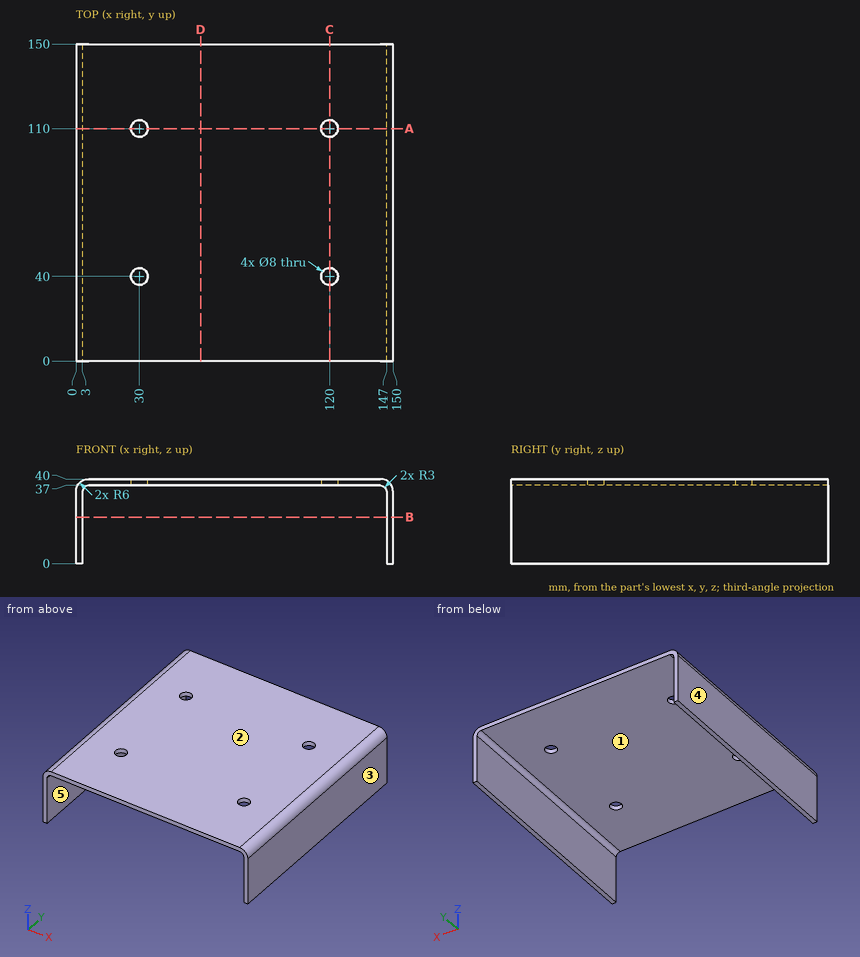
Print and shaded views of the part. All mm, measured from the part's lowest x, y and z. A direction names the side the tool comes from. Give positions to 0.01 mm unless a question says otherwise; leave off trailing zeros. Loops run counter-clockwise (first coordinate to the right, second up) from the corner with the lowest first, then second, coordinate; pieces in that order, holes last. Notation, with made-up numbers: (-13.75, 24) - (-2.75, 24) arc R29 cw to (-2.75, 61) - close; hole circle Ø3 at (35.25, 44.25). An arc over 180 degrees is marked (long way). One line per item, written item: value. Start each with the question number.
1. Which spindle directions (+Z, -Z, +X, -X, +Y, -Y) get a long thin tool onto all of the face, cutting with end or side? Do the marked faces 4 and 5. Say none if no direction does.
2. Pin check, flat tips, straight feed: pin 1 (6.5 mm diameter, centred on x = 30, y = 110, fed in from +Z) (3 decimals); pin 2 (3 mm diameter, centred on x = 113.5, y = 115, fed in from -Z). Stop position of each tip, or through.
3. Slice it at B-B (z = 22). List the corners of the cut face in (x, y).
4. Probe L1, parallel to Y at x = 120, z = 38.5; L2, parallel to X at y = 26.5, z = 6; L3, parallel to X at y = 110, z = 37.65. List the from-to ranges inside material, lowest first. Write a range as from..to.
5. Slice it at D-D (x = 59). List the corners of the cut face in (y, z), plus the area to 3 significant figures.
6. Slice it at C-C (x = 120). List the corners of the cut face in (y, z).
7. Pull direction X, two halves, no side cores. Call the marked faces 1, 2 and 3: pulls with the +X half, pulls with the -X half, needs draft (parallel to the pull), parting line crosses it, or undercut.
8. Slice it at A-A (y = 110). List the corners of the cut face in (x, z).
Solution:
1. face 4: +Z, -Z, -X, +Y, -Y
1. face 5: -Z, +Y, -Y
2. pin 1: passes through
2. pin 2: stops at z = 37
3. outline: (0, 0) - (3, 0) - (3, 150) - (0, 150) - close; (147, 0) - (150, 0) - (150, 150) - (147, 150) - close
4. L1: y = 0..36, 44..106, 114..150
4. L2: x = 0..3, 147..150
4. L3: x = 1.24..26, 34..116, 124..148.76
5. outline: (0, 37) - (150, 37) - (150, 40) - (0, 40) - close
5. area: 450 mm^2
6. outline: (0, 37) - (36, 37) - (36, 40) - (0, 40) - close; (44, 37) - (106, 37) - (106, 40) - (44, 40) - close; (114, 37) - (150, 37) - (150, 40) - (114, 40) - close
7. face 1: undercut
7. face 2: needs draft
7. face 3: pulls with the +X half
8. outline: (0, 0) - (3, 0) - (3, 34) arc R3 cw to (6, 37) - (26, 37) - (26, 40) - (6, 40) arc R6 ccw to (0, 34) - close; (34, 37) - (116, 37) - (116, 40) - (34, 40) - close; (124, 37) - (144, 37) arc R3 cw to (147, 34) - (147, 0) - (150, 0) - (150, 34) arc R6 ccw to (144, 40) - (124, 40) - close
